Source: CAD feature listing. Evaluate the final solid. Frame: model axes, mm. Face numbers are marked on the shaded views. Round coordinates to 2 decimals unless told otherwise and drop trailing zeros. Write each loop counter-clockwise with the first axis right and the second up, starting at its lowest first coordinate (ties: lowest second). Pieces come first, ordered by that corner, then holes. Notation, with made-up numbers: M -25,85 L 31,85 A23 ccw 31,112 Z; hole C -23,14.25 d1. An arc over 180 degrees is marked long. Answer in a Markdown table with one row per item. Add a question column.
Item 1: Cut plane B-B on z = 0. Return loops of the section in (x, y), and give its area (3 significant figures).
Item 2: Mould query, pull axis X, two halves, no side actions, for the marked faces 1 and 2. Classes: released by +X, released by -X, zero draft, split by the parting line, or undercut.
Item 3: Contact query for flat-ended pins moving along their axis: pin 1 (1 mm diameter, centred on x = -1.5, z = -10.5, fed in from +Y); pin 2 (9.5 mm diameter, centred on x = -13.1, z = 0, fed in from +Y); pin 3 (1 mm diameter, centred on x = -11.5, y = 4, fed in from +Z); pin 4 (0.5 mm diameter, centred on x = -9.5, y = 0.5, fed in from +Z). Output: stop coordinate, or through.
Item 4: Material intervals for probe 1 along X at (y, z) = (2.5, -15); probe 2 along X at (y, z) = (0.55, 0); probe 3 along Z at (x, y) = (-16.5, 2.3), sorted ascending.
Item 5: Cut plane D-D on y = 0.5. Give the number of separate pieces and of enclosed holes in the cut face, and give its area (3 significant figures).
Item 6: Cut plane A-A on y = 2.6. Return loops of the section in (x, z), and give its area (3 significant figures).
Item 7: Cut plane C-C on x = 0. Return loops of the section in (y, z), and give its area (3 significant figures).
from build123d import *

# Parameters (mm, degrees)
SKETCH1_R           = 3.65
SKETCH1_R_2         = 1.75
BOSS_EXTRUDE1_DEPTH = 1
SKETCH2_R           = 3.25
SKETCH2_R_2         = 1.75
BOSS_EXTRUDE2_DEPTH = 3.5


with BuildPart() as part:
    # Sketch1 → Boss-Extrude1 (new body)
    with BuildSketch(Plane(origin=(0, 0, 0), x_dir=(1, 0, 0), z_dir=(0, 1, 0))):
        with BuildLine():
            Line((5.410568808, -5.6), (13.1, -5.6))
            ThreePointArc((13.1, -5.6), (18.7, 0), (13.1, 5.6))
            Line((13.1, 5.6), (5.410568808, 5.6))
            add(Edge.make_bspline(
                [(15, 11.75), (9.437012866, 9.684618997), (5.410568808, 5.6)],
                knots=[0, 0, 0, 0.823024689, 0.823024689, 0.823024689], degree=2))
            ThreePointArc((15, 11.75), (18.002608481, 16.243721155), (12.701902961, 17.298097039))
            add(Edge.make_bspline(
                [(12.701902961, 17.298097039), (8.967561343, 14.947817201), (5.535660126, 12.253556278)],
                knots=[0, 0, 0, 0.409026758, 0.409026758, 0.409026758], degree=2))
            ThreePointArc((5.535660126, 12.253556278), (0, 18.7), (-5.535660126, 12.253556278))
            add(Edge.make_bspline(
                [(-5.535660126, 12.253556278), (-8.967561343, 14.947817201), (-12.701902961, 17.298097039)],
                knots=[0.751545437, 0.751545437, 0.751545437, 1.160572194, 1.160572194, 1.160572194], degree=2))
            ThreePointArc((-12.701902961, 17.298097039), (-18.002608481, 16.243721155), (-15, 11.75))
            add(Edge.make_bspline(
                [(-15, 11.75), (-9.437012866, 9.684618997), (-5.410568808, 5.6)],
                knots=[0, 0, 0, 0.823024689, 0.823024689, 0.823024689], degree=2))
            Line((-5.410568808, 5.6), (-13.1, 5.6))
            ThreePointArc((-13.1, 5.6), (-18.7, 0), (-13.1, -5.6))
            Line((-13.1, -5.6), (-5.410568808, -5.6))
            add(Edge.make_bspline(
                [(-15, -11.75), (-9.437012866, -9.684618997), (-5.410568808, -5.6)],
                knots=[0, 0, 0, 0.823024689, 0.823024689, 0.823024689], degree=2))
            ThreePointArc((-15, -11.75), (-18.002608481, -16.243721155), (-12.701902961, -17.298097039))
            add(Edge.make_bspline(
                [(-12.701902961, -17.298097039), (-8.967561343, -14.947817201), (-5.535660126, -12.253556278)],
                knots=[0, 0, 0, 0.409026758, 0.409026758, 0.409026758], degree=2))
            ThreePointArc((-5.535660126, -12.253556278), (0, -18.7), (5.535660126, -12.253556278))
            add(Edge.make_bspline(
                [(5.535660126, -12.253556278), (8.967561343, -14.947817201), (12.701902961, -17.298097039)],
                knots=[0.751545437, 0.751545437, 0.751545437, 1.160572194, 1.160572194, 1.160572194], degree=2))
            ThreePointArc((12.701902961, -17.298097039), (18.002608481, -16.243721155), (15, -11.75))
            add(Edge.make_bspline(
                [(15, -11.75), (9.437012866, -9.684618997), (5.410568808, -5.6)],
                knots=[0, 0, 0, 0.823024689, 0.823024689, 0.823024689], degree=2))
        make_face()
        with Locations(Location((0, 13.1, 0), (0, 0, 270))):
            Circle(SKETCH1_R, mode=Mode.SUBTRACT)
        with Locations(Location((0, -13.1, 0), (0, 0, 270))):
            Circle(SKETCH1_R, mode=Mode.SUBTRACT)
        with Locations(Location((13.1, 0, 0), (0, 0, 270))):
            Circle(SKETCH1_R, mode=Mode.SUBTRACT)
        with Locations(Location((15, 15, 0), (0, 0, 270))):
            Circle(SKETCH1_R_2, mode=Mode.SUBTRACT)
        with Locations(Location((-13.1, 0, 0), (0, 0, 270))):
            Circle(SKETCH1_R, mode=Mode.SUBTRACT)
        with Locations(Location((-15, 15, 0), (0, 0, 270))):
            Circle(SKETCH1_R_2, mode=Mode.SUBTRACT)
        with Locations(Location((15, -15, 0), (0, 0, 270))):
            Circle(SKETCH1_R_2, mode=Mode.SUBTRACT)
        with Locations(Location((-15, -15, 0), (0, 0, 270))):
            Circle(SKETCH1_R_2, mode=Mode.SUBTRACT)
    extrude(amount=BOSS_EXTRUDE1_DEPTH)

    # Sketch2 → Boss-Extrude2 (add)
    # profile 1 of 4: a face of its own
    with BuildSketch(Plane(origin=(0, 1, 0), x_dir=(1, 0, 0), z_dir=(0, 1, 0))):
        with Locations(Location((-15, 15, 0), (0, 0, 270))):
            Circle(SKETCH2_R)
        with Locations(Location((-15, 15, 0), (0, 0, 270))):
            Circle(SKETCH2_R_2, mode=Mode.SUBTRACT)
    # profile 2 of 4: a face of its own
    with BuildSketch(Plane(origin=(0, 1, 0), x_dir=(1, 0, 0), z_dir=(0, 1, 0))):
        with Locations(Location((15, 15, 0), (0, 0, 270))):
            Circle(SKETCH2_R)
        with Locations(Location((15, 15, 0), (0, 0, 270))):
            Circle(SKETCH2_R_2, mode=Mode.SUBTRACT)
    # profile 3 of 4: a face of its own
    with BuildSketch(Plane(origin=(0, 1, 0), x_dir=(1, 0, 0), z_dir=(0, 1, 0))):
        with Locations(Location((15, -15, 0), (0, 0, 90))):
            Circle(SKETCH2_R)
        with Locations(Location((15, -15, 0), (0, 0, 270))):
            Circle(SKETCH2_R_2, mode=Mode.SUBTRACT)
    # profile 4 of 4: a face of its own
    with BuildSketch(Plane(origin=(0, 1, 0), x_dir=(1, 0, 0), z_dir=(0, 1, 0))):
        with Locations(Location((-15, -15, 0), (0, 0, 90))):
            Circle(SKETCH2_R)
        with Locations(Location((-15, -15, 0), (0, 0, 270))):
            Circle(SKETCH2_R_2, mode=Mode.SUBTRACT)
    extrude(amount=BOSS_EXTRUDE2_DEPTH)


solid = part.part
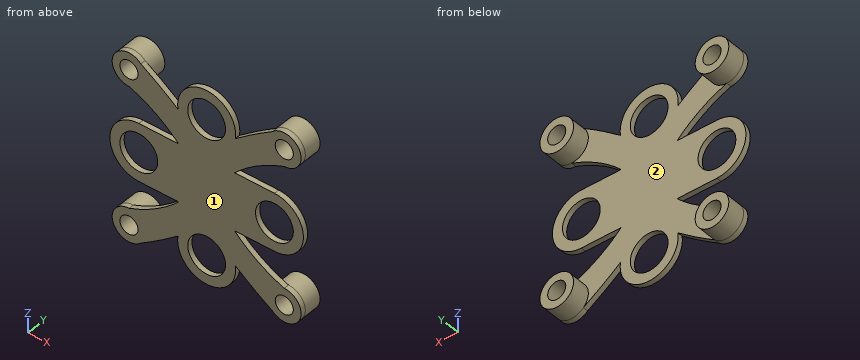
Results below:
| question | item | result |
|---|---|---|
| 1 | outline | M -18.7,0 L -16.75,0 L -16.75,1 L -18.7,1 Z; M -9.45,0 L 9.45,0 L 9.45,1 L -9.45,1 Z; M 16.75,0 L 18.7,0 L 18.7,1 L 16.75,1 Z |
| 1 | area | 22.8 mm2 |
| 2 | face 1 | zero draft |
| 2 | face 2 | undercut |
| 3 | pin 1 | through |
| 3 | pin 2 | y = 1 |
| 3 | pin 3 | z = 16.25 |
| 3 | pin 4 | z = 15.35 |
| 4 | probe 1 | -18.25 to -16.75, -13.25 to -11.75, 11.75 to 13.25, 16.75 to 18.25 |
| 4 | probe 2 | -18.7 to -16.75, -9.45 to 9.45, 16.75 to 18.7 |
| 4 | probe 3 | -17.88 to -15.9, -14.1 to -12.12, 12.12 to 14.1, 15.9 to 17.88 |
| 5 | separate pieces | 1 |
| 5 | enclosed holes | 8 |
| 5 | area | 759 mm2 |
| 6 | outline | C -15,-15 d6.5; C -15,15 d6.5; C 15,-15 d6.5; C 15,15 d6.5; hole C -15,-15 d3.5; hole C -15,15 d3.5; hole C 15,-15 d3.5; hole C 15,15 d3.5 |
| 6 | area | 94.2 mm2 |
| 7 | outline | M 0,-18.7 L 1,-18.7 L 1,-16.75 L 0,-16.75 Z; M 0,-9.45 L 1,-9.45 L 1,9.45 L 0,9.45 Z; M 0,16.75 L 1,16.75 L 1,18.7 L 0,18.7 Z |
| 7 | area | 22.8 mm2 |
